from build123d import *

# Parameters (mm, degrees)
MAINBASESKETCH_W                = 7.9
MAINBASESKETCH_H                = 12.8
MAINBASEEXTRUDE_DEPTH           = 7.9
STUDSSKETCH_R                   = 2.4
STUDSEXTRUDE_DEPTH              = 1.6
STUDSPATTERN_COUNT              = 2
STUDSPATTERN_PITCH              = 8
MAINBASESHELL_T                 = -1.2
SLIMYELLOWUNDEREXT_START        = -0.2
SLIMYELLOWUNDEREXT_DEPTH        = 11.6
ZIGZAGSKETCH_W                  = 7.9
ZIGZAGSKETCH_H                  = 3.2
ZIGZAGBLUEEXT_DEPTH             = 15.8
LPATTERN1_COUNT                 = 2
LPATTERN1_PITCH                 = 8
LPATTERN1_COPY_1_SKETCH_R       = 2.4
LPATTERN1_COPY_1_DEPTH          = 1.6
ZIGZAGSTUDSKETCH_R              = 2.4
ADDEDSTUDSZIGZAG_DEPTH          = 1.6
CUTUSEDASSHELLSKETCH_W          = 6.71130504
CUTUSEDASSHELLSKETCH_H          = 13.400349982
CUTUSEDASSHELL_DEPTH            = 2.4
ZIGZAGUNDERSTUDSSKETCH_R        = 1.2
ZIGZAGUNDERSTUDHOLES_DEPTH      = 1.7
ZIGZAGUNDERSEMICIRCLEEXT_START  = -0.2
ZIGZAGUNDERSEMICIRCLEEXT_DEPTH  = 1.6
CUTUSEDASSHELLSKETCH2_W         = 6.7
CUTUSEDASSHELLSKETCH2_H         = 13.4
CUTUSEDASSHELL2_DEPTH           = 2.4
ZIGZAGUNDERSEMICEXT2_START      = -0.2
ZIGZAGUNDERSEMICEXT2_DEPTH      = 1.6
ZIGZAGINSIDECORNER1_R           = 1
ZIGZAGINSIDECORNER2_R           = 1
ZIGZAGUNDERSTUDSKETCH2_R        = 1.2
CUT_EXTRUDE1_DEPTH              = 1.7
RECTANGULARUNDEREXTRUDES1_START = -0.2
RECTANGULAREXTSKETCH_W          = 1.100347559
RECTANGULAREXTSKETCH_H          = 0.995198726
RECTANGULARUNDEREXTRUDES1_DEPTH = 1.5
RECTANGULARUNDEREXTRUDES2_START = -0.2
RECTANGULARUNDEREXTSKETCH2_W    = 1.105292793
RECTANGULARUNDEREXTSKETCH2_H    = 0.995198726
RECTANGULARUNDEREXTRUDES2_DEPTH = 1.5


with BuildPart() as part:
    # MainBaseSketch → MainBaseExtrude (new, symmetric)
    with BuildSketch(Plane.XY):
        with Locations((4.631967213, 6.4)):
            Rectangle(MAINBASESKETCH_W, MAINBASESKETCH_H)
    extrude(amount=MAINBASEEXTRUDE_DEPTH, both=True)

    # StudsSketch → StudsExtrude (add)
    with BuildSketch(Plane(origin=(0, 12.8, 0), x_dir=(1, 0, 0), z_dir=(0, 1, 0))):
        with Locations(Location((4.581967213, 4, 0), (0, 0, 90))):
            Circle(STUDSSKETCH_R)
    studsextrude = extrude(amount=STUDSEXTRUDE_DEPTH)

    # StudsPattern: StudsExtrude ×2
    with Locations(*[(0, 0, i * STUDSPATTERN_PITCH) for i in range(1, STUDSPATTERN_COUNT)]):
        add(studsextrude)

    # MainBaseShell
    mainbaseshell_openings = [part.faces().sort_by_distance(p)[0] for p in [
        (4.631967213, 0, 0),
    ]]
    offset(amount=MAINBASESHELL_T, openings=mainbaseshell_openings, kind=Kind.INTERSECTION)

    # SlimYellowUnderExtSketch → SlimYellowUnderExt (add)
    with BuildSketch(Plane.XZ.offset(-11.6).offset(SLIMYELLOWUNDEREXT_START)):
        Polygon((1.881967213, 1.952811318), (1.881967213, 2.947188682), (2.384104441, 2.947188682), (2.882626102, 2.45), (2.384104441, 1.952811318), align=None)
        Polygon((6.381308324, 2.45), (6.879829986, 2.947188682), (7.381967213, 2.947188682), (7.381967213, 1.952811318), (6.879829986, 1.952811318), align=None)
        Polygon((1.881967213, -1.952811318), (2.384104441, -1.952811318), (2.882626102, -2.45), (2.384104441, -2.947188682), (1.881967213, -2.947188682), align=None)
        Polygon((7.381967213, -1.952811318), (7.381967213, -2.947188682), (6.879829986, -2.947188682), (6.381308324, -2.45), (6.879829986, -1.952811318), align=None)
    extrude(amount=SLIMYELLOWUNDEREXT_DEPTH)

    # ZigZagSketch → ZIGZAGBlueExt (add)
    with BuildSketch(Plane.XY.offset(7.9)):
        with Locations((-3.268032787, 11.2)):
            Rectangle(ZIGZAGSKETCH_W, ZIGZAGSKETCH_H)
        with Locations((12.531967213, 1.6)):
            Rectangle(ZIGZAGSKETCH_W, ZIGZAGSKETCH_H)
    extrude(amount=-ZIGZAGBLUEEXT_DEPTH)

    # LPattern1: StudsExtrude ×2
    with Locations(*[(-i * LPATTERN1_PITCH, 0, 0) for i in range(1, LPATTERN1_COUNT)]):
        add(studsextrude)

    # LPattern1 copy 1 sketch → LPattern1 copy 1 (add)
    with BuildSketch(Plane(origin=(-8, 12.8, 8), x_dir=(1, 0, 0), z_dir=(0, 1, 0))):
        with Locations(Location((4.581967213, 4, 0), (0, 0, 90))):
            Circle(LPATTERN1_COPY_1_SKETCH_R)
    extrude(amount=LPATTERN1_COPY_1_DEPTH)

    # ZigZagStudSketch → AddedStudsZigZag (add)
    with BuildSketch(Plane(origin=(0, 3.2, 0), x_dir=(1, 0, 0), z_dir=(0, 1, 0))):
        with Locations(Location((12.531967213, 3.95, 0), (0, 0, 270))):
            Circle(ZIGZAGSTUDSKETCH_R)
        with Locations(Location((12.531967213, -3.95, 0), (0, 0, 90))):
            Circle(ZIGZAGSTUDSKETCH_R)
    extrude(amount=ADDEDSTUDSZIGZAG_DEPTH)

    # CutUsedAsShellSketch → CutUsedasShell (cut)
    with BuildSketch(Plane.XZ):
        with Locations((11.948290767, 0)):
            Rectangle(CUTUSEDASSHELLSKETCH_W, CUTUSEDASSHELLSKETCH_H)
    extrude(amount=-CUTUSEDASSHELL_DEPTH, mode=Mode.SUBTRACT)

    # ZigZagUnderStudsSketch → ZigZagUnderStudHoles (cut)
    with BuildSketch(Plane.XZ.offset(-2.4)):
        with Locations(Location((13.103943287, 4, 0), (0, 0, 270))):
            Circle(ZIGZAGUNDERSTUDSSKETCH_R)
        with Locations(Location((13.103943287, -4, 0), (0, 0, 90))):
            Circle(ZIGZAGUNDERSTUDSSKETCH_R)
    extrude(amount=-ZIGZAGUNDERSTUDHOLES_DEPTH, mode=Mode.SUBTRACT)

    # ZigZAgUNderSemiCSketch → ZigZagUnderSemiCircleExt (add)
    with BuildSketch(Plane.XZ.offset(-2.4).offset(ZIGZAGUNDERSEMICIRCLEEXT_START)):
        with BuildLine():
            ThreePointArc((8.592638247, -3.25057639), (11.595624855, -0.104008885), (8.592638247, 3.04255862))
            Line((8.592638247, 3.04255862), (8.592638247, 2.4))
            ThreePointArc((8.592638247, 2.4), (10.992638247, 0), (8.592638247, -2.4))
            Line((8.592638247, -2.4), (8.592638247, -2.40057639))
            Line((8.592638247, -2.40057639), (8.592638247, -3.25057639))
        make_face()
    extrude(amount=ZIGZAGUNDERSEMICIRCLEEXT_DEPTH)

    # CutUsedAsShellSketch2 → CutUsedAsShell2 (cut)
    with BuildSketch(Plane.XZ.offset(-9.6)):
        with Locations((-2.668032787, 0)):
            Rectangle(CUTUSEDASSHELLSKETCH2_W, CUTUSEDASSHELLSKETCH2_H)
    extrude(amount=-CUTUSEDASSHELL2_DEPTH, mode=Mode.SUBTRACT)

    # ZigZagUnderSemiCExtSketch → ZigZagUnderSemiCExt2 (add)
    with BuildSketch(Plane.XZ.offset(-12).offset(ZIGZAGUNDERSEMICEXT2_START)):
        with BuildLine():
            Line((0.681967213, -3.12), (0.681967213, -2.45))
            ThreePointArc((0.681967213, -2.45), (-1.768032787, 0), (0.681967213, 2.45))
            Line((0.681967213, 2.45), (0.681967213, 3.12))
            ThreePointArc((0.681967213, 3.12), (-2.438032787, 0), (0.681967213, -3.12))
        make_face()
    extrude(amount=ZIGZAGUNDERSEMICEXT2_DEPTH)

    # ZigZagInsideCorner1
    zigzaginsidecorner1_edges = [part.edges().sort_by_distance(p)[0] for p in [
        (8.592638247, 1.2, -6.700174991),
        (8.592638247, 1.2, 6.700174991),
    ]]
    fillet(zigzaginsidecorner1_edges, radius=ZIGZAGINSIDECORNER1_R)

    # ZigZagInsideCorner2
    zigzaginsidecorner2_edges = [part.edges().sort_by_distance(p)[0] for p in [
        (0.681967213, 10.8, -6.7),
        (0.681967213, 10.8, 6.7),
    ]]
    fillet(zigzaginsidecorner2_edges, radius=ZIGZAGINSIDECORNER2_R)

    # ZigZagUnderStudSketch2 → Cut-Extrude1 (cut)
    with BuildSketch(Plane.XZ.offset(-12)):
        with Locations((-3.818032787, 4)):
            Circle(ZIGZAGUNDERSTUDSKETCH2_R)
        with Locations((-3.818032787, -4)):
            Circle(ZIGZAGUNDERSTUDSKETCH2_R)
    extrude(amount=-CUT_EXTRUDE1_DEPTH, mode=Mode.SUBTRACT)

    # RectangularExtSketch → RectangularUnderExtrudes1 (add)
    with BuildSketch(Plane.XZ.offset(-12).offset(RECTANGULARUNDEREXTRUDES1_START)):
        with Locations((0.131793434, 4.747212315)):
            Rectangle(RECTANGULAREXTSKETCH_W, RECTANGULAREXTSKETCH_H)
        with Locations((0.131793434, -4.747212315)):
            Rectangle(RECTANGULAREXTSKETCH_W, RECTANGULAREXTSKETCH_H)
    extrude(amount=RECTANGULARUNDEREXTRUDES1_DEPTH)

    # RectangularUnderExtSketch2 → RectangularUnderExtrudes2 (add)
    with BuildSketch(Plane.XZ.offset(-2.4).offset(RECTANGULARUNDEREXTRUDES2_START)):
        with Locations((9.153257665, 4.747212315)):
            Rectangle(RECTANGULARUNDEREXTSKETCH2_W, RECTANGULARUNDEREXTSKETCH2_H)
        with Locations((9.153257665, -4.747212315)):
            Rectangle(RECTANGULARUNDEREXTSKETCH2_W, RECTANGULARUNDEREXTSKETCH2_H)
    extrude(amount=RECTANGULARUNDEREXTRUDES2_DEPTH)


solid = part.part
Model file for the job. Use its own axes, mm. A direction names the side the tool comes from. Coordinates: 2 decimals unless noted, no trailing zeros. Write each loop counter-clockwise with the first axis right and the second up, starting at its lowest first coordinate (ties: lowest second). Pieces come first, ordered by that corner, then holes. Notation, with made-up numbers: (71, -9.5) - (77, -9.5) arc R35 cw to (77, 24.5) - close; hole circle Ø4 at (-20, -11.75). An arc over 180 degrees is marked (long way). Write each question's results on one line, items separated by ' | '. Start each with the question number.
1) Cut at A-A (y = 5.5). Write the cut outline in (x, z), then the cut area to 3 significant figures.
2) Cut at C-C (z = 1.25). Write the cut outline in (x, y), then the cut area to 3 significant figures.
3) Cut at D-D (x = 1.5). Write the cut outline in (y, z).
4) Mould opens along X. For faces 1 (the face through (5, 14.4, -4)), 2 (the face through (9, 2, -4.25)), 3 (the face through (-7.218, 11, 0)) say: pulls with the +X half, pulls with the -X half, needs draft (parallel to the pull), parting line crosses it, or undercut.
5) Flat gauge pins, fed straight in: P1, Ø1.9, axis at y = 1, z = -0.5, coming from the -X side; P2, Ø1, axis at x = 4.5, z = -3.5, coming from the -Y side; P3, Ø6, axis at y = 6.5, z = 2, coming from the +X side; P4, Ø1.1, axis at x = 0.5, z = -5, coming from the -Y side. Where does each tip first touch, or does it go through?
6) Probe line 1 along X through (y, z) = (3.7, -4); line 2 along X through (y, z) = (2.8, -4); line 3 along Z through (x, y) = (6, 1.75). List the from-to ranges inside material, lowest first. Write a range as from..to.
7) Cut at B-B (y = 3.75). Count the separate pieces of the cut face and the enclosed holes in it, then the cut area to 3 significant figures.
8) 3-axis set-ups, long thin cutter, end or side, ignore diameter. For faces 4 (the face through (12, 3.2, 0)), 5 (the face through (5, 14.4, 4)), 6 (the face through (8.582, 8, 0)), 7 (the face through (0, 10.7, -5)): which of +Z, -Z, +X, -X, +Y, -Y reach the whole face in a straight line?
Returned:
1) outline: (0.68, -7.9) - (8.58, -7.9) - (8.58, 7.9) - (0.68, 7.9) - close; hole (1.88, -6.7) - (7.38, -6.7) - (7.38, -2.95) - (6.88, -2.95) - (6.38, -2.45) - (6.88, -1.95) - (7.38, -1.95) - (7.38, 1.95) - (6.88, 1.95) - (6.38, 2.45) - (6.88, 2.95) - (7.38, 2.95) - (7.38, 6.7) - (1.88, 6.7) - (1.88, 2.95) - (2.38, 2.95) - (2.88, 2.45) - (2.38, 1.95) - (1.88, 1.95) - (1.88, -1.95) - (2.38, -1.95) - (2.88, -2.45) - (2.38, -2.95) - (1.88, -2.95) - close | area: 54.1 mm^2
2) outline: (-7.22, 9.6) - (-6.02, 9.6) - (-6.02, 12) - (-2.18, 12) - (-2.18, 10.6) - (-1.43, 10.6) - (-1.43, 12) - (0.68, 12) - (0.68, 0) - (1.88, 0) - (1.88, 11.6) - (7.38, 11.6) - (7.38, 0) - (8.59, 0) - (8.59, 2.4) - (10.64, 2.4) - (10.64, 1) - (11.29, 1) - (11.29, 2.4) - (15.3, 2.4) - (15.3, 0) - (16.48, 0) - (16.48, 3.2) - (8.58, 3.2) - (8.58, 12.8) - (-7.22, 12.8) - close | area: 57.7 mm^2
3) outline: (0, -7.9) - (12.8, -7.9) - (12.8, 7.9) - (0, 7.9) - close
4) face 1: needs draft | face 2: undercut | face 3: pulls with the -X half
5) P1: x = 0.68 | P2: y = 13.2 | P3: x = 14.93 | P4: y = 0
6) line 1: 0.68..1.88, 7.38..8.58, 10.13..11.9, 14.3..14.93 | line 2: 0.68..1.88, 7.38..11.9, 14.3..16.48 | line 3: -7.9..-6.7, 6.7..7.9
7) separate pieces: 3 | enclosed holes: 3 | area: 81.3 mm^2
8) face 4: +Y | face 5: +Z, -Z, +X, -X, +Y | face 6: +Z, -Z, +Y | face 7: -Y
